Autodesk Inventor part; units mm, degrees
ref_plane "YZ Plane" through (0, 0, 0) normal (1, 0, 0) x (0, 1, 0)
ref_plane "XZ Plane" through (0, 0, 0) normal (0, 1, 0) x (-1, 0, 0)
ref_plane "XY Plane" through (0, 0, 0) normal (0, 0, 1) x (1, 0, 0)
sketch "Sketch2" plane through (0, 0, 0) normal (0, 0, 1) x (1, 0, 0)
  line L0 (-36.8686, 26.7016) -> (-30.1114, 30.7457)
  line L1 (-30.1114, 30.7457) -> (-23.2304, 26.9158)
  line L2 (-23.2304, 26.9158) -> (-23.1068, 19.0418)
  line L3 (-23.1068, 19.0418) -> (-29.864, 14.9977)
  line L4 (-29.864, 14.9977) -> (-36.7449, 18.8276)
  line L5 (-36.7449, 18.8276) -> (-36.8686, 26.7016)
  line L6 (-111.0137, 35.5717) -> (-17.2877, 35.5717)
  line L7 (-17.2877, 35.5717) -> (-17.2877, -24.1183)
  line L8 (-17.2877, -24.1183) -> (-111.0137, -24.1183)
  line L9 (-111.0137, -24.1183) -> (-111.0137, 35.5717)
  line L10 (-101.137, 28.7391) -> (-70.6621, 28.7391)
  line L11 (-70.6621, 28.7391) -> (-70.6621, -18.2509)
  line L12 (-70.6621, -18.2509) -> (-101.137, -18.2509)
  line L13 (-101.137, -18.2509) -> (-101.137, 28.7391)
  point P0 (0, 0)
  point P1 (-29.9877, 22.8717)
  dimension "d1" = 7.874
  dimension "d3" = 59.69
  dimension "d5" = 12.7
  dimension "d6" = 93.726
  dimension "d39" = 46.99
  dimension "d41" = 6.8326
  dimension "d42" = 5.8674
  dimension "d43" = 12.7
extrude "Extrusion1" add sketch "Sketch2" along normal blind 6.35 contours L6 L7 L8 L9 | L10 L11 L12 L13
sketch "Sketch3" plane through (0, 0, 6.35) normal (0, 0, 1) x (1, 0, 0)
  circle A0 centre (-107.8387, 30.4917) radius 1.905
  line L0 (-17.2877, 35.5717) -> (-111.0137, 35.5717)
  line L1 (-111.0137, 35.5717) -> (-111.0137, -24.1183)
  circle A1 centre (-107.8387, 20.3317) radius 1.905
  circle A2 centre (-107.8387, -10.1483) radius 1.905
  circle A3 centre (-107.8387, -20.3083) radius 1.905
  line L2 (-111.0137, -24.1183) -> (-17.2877, -24.1183)
  circle A4 centre (-107.8387, 10.1717) radius 1.905
  circle A5 centre (-107.8387, 0.0117) radius 1.905
  point P0 (0, 0)
  dimension "d9" = 3.81
  dimension "d10" = 5.08
  dimension "d11" = 3.175
  dimension "d13" = 3.81
  dimension "d14" = 3.81
  dimension "d15" = 3.81
  dimension "d17" = 3.175
  dimension "d18" = 3.175
  dimension "d19" = 3.175
  dimension "d21" = 10.16
  dimension "d24" = 3.81
  dimension "d25" = 3.81
  dimension "d26" = 3.175
  dimension "d27" = 3.175
  dimension "d28" = 10.16
  dimension "d29" = 10.16
  dimension "d33" = 10.16
  dimension "d44" = 10.16
extrude "Extrusion2" cut sketch "Sketch3" against normal blind 3.81
sketch "Sketch4" plane through (0, 0, 6.35) normal (0, 0, 1) x (1, 0, 0)
  line L0 (-17.2877, 35.5717) -> (-111.0137, 35.5717)
  line L1 (-72.9137, 35.5717) -> (-60.2137, 35.5717)
  line L2 (-60.2137, 35.5717) -> (-60.2137, 35.0891)
  line L3 (-60.2137, 35.0891) -> (-72.9137, 35.0891)
  line L4 (-72.9137, 35.0891) -> (-72.9137, 35.5717)
  line L5 (-111.0137, -24.1183) -> (-17.2877, -24.1183)
  line L6 (-111.0137, 35.5717) -> (-111.0137, -24.1183)
  line L7 (-72.9137, 35.5717) -> (-60.2137, 35.5717)
  line L8 (-60.2137, 35.5717) -> (-60.2137, 28.7391)
  line L9 (-60.2137, 28.7391) -> (-72.9137, 28.7391)
  line L10 (-72.9137, 28.7391) -> (-72.9137, 35.5717)
  line L11 (-69.1037, -24.1183) -> (-81.8037, -24.1183)
  line L12 (-81.8037, -24.1183) -> (-81.8037, -18.1493)
  line L13 (-81.8037, -18.1493) -> (-69.1037, -18.1493)
  line L14 (-69.1037, -18.1493) -> (-69.1037, -24.1183)
  point P0 (0, 0)
  dimension "d34" = 59.2074
  dimension "d35" = 12.7
  dimension "d36" = 38.1
  dimension "d45" = 6.8326
  dimension "d46" = 12.7
  dimension "d47" = 5.969
  dimension "d48" = 29.21
extrude "Extrusion3" add sketch "Sketch4" along normal blind 6.35
properties part number "polyhexpart"
Could you check a few things on this model? Use its own coordinates, in mm. A direction names the side the tool comes from. Round coordinates to 2 decimals unless told otherwise and drop trailing zeros. Write each loop counter-clockwise with the first axis right and the second up, starting at its lowest first coordinate (ties: lowest second). Pieces come first, ordered by that corner, then holes. Notation, with made-up numbers: M 69,27 L 104,27 A15 ccw 104,33 Z; hole C 0,-15.75 d5. An arc over 180 degrees is marked long. Answer in a Markdown table with one row per item. Add a question column.
Q1. Imagine slicing it at B-B (x = -70.5). Please give me the cut outline in (y, z).
Q2. Will these pins go through, and if not, where does the flat tip stop? pin 1 Ø3 at (x, y) = (-34.5, 18.5) entering from +Z; pin 2 Ø4.5 at (x, y) = (-107.84, -20.31) entering from -Z; pin 3 Ø7 at (x, z) = (-64.5, 10.5) entering from -Y; pin 4 Ø1.9 at (x, y) = (-108, -11) entering from +Z.
Q3. Imagine slicing it at D-D (z = 3.5). Please give me the cut outline in (x, y) (3 decimals), then the cut area to 3 significant figures.
Q4. Imagine slicing it at C-C (x = -25). Please give me the cut outline in (y, z), then the cut area to 3 significant figures.
Q5. On a 3-axis mill with a long thin cutter (end or side, diameter ignored), from which of +Z, -Z, +X, -X, +Y, -Y can I reach the whole of each face in a straight line? I mean faces 1 (the flat face through (-69.104, -21, 9)), 2 (the cylindrical face through (-106.02, 10.74, 4.47)), 3 (the flat face through (-76, -18.149, 9)). Say none if no direction works.
Q6. If I drill on line 1 (X direction, y = 10, z = 5.5); line 2 (X direction, y = 25.5, z = 3.25); line 3 (X direction, y = 20, z = 3), over which ranges is the centre line in solid material (lowest first)? Write a range as from..to.
Q7. Imagine slicing it at A-A (z = 8.25). Please give me the cut outline in (x, y).
Q8. If we mould it in two halves opening along Y, with no side actions, what happens to faces 4 (the flat face through (-65, 35.572, 3)), 5 (the flat face through (-108, 0, 2.54)), 6 (the flat face through (-72.914, 32, 9))? For each: +Y half, -Y half, draft (parallel to the pull), parting line (faces both ways), or undercut.
Values:
| question | item | result |
|---|---|---|
| 1 | outline | M -24.12,0 L 35.57,0 L 35.57,12.7 L 28.74,12.7 L 28.74,6.35 L -18.15,6.35 L -18.15,12.7 L -24.12,12.7 Z |
| 2 | pin 1 | z = 6.35 |
| 2 | pin 2 | z = 0 |
| 2 | pin 3 | y = 28.74 |
| 2 | pin 4 | z = 2.54 |
| 3 | outline | M -111.014,-24.118 L -17.288,-24.118 L -17.288,35.572 L -111.014,35.572 Z; hole C -107.839,-20.308 d3.81; hole C -107.839,-10.148 d3.81; hole C -107.839,0.012 d3.81; hole C -107.839,10.172 d3.81; hole C -107.839,20.332 d3.81; hole C -107.839,30.492 d3.81; hole M -36.869,26.702 L -36.745,18.828 L -29.864,14.998 L -23.107,19.042 L -23.23,26.916 L -30.111,30.746 Z |
| 3 | area | 5,360 mm^2 |
| 4 | outline | M -24.12,0 L 17.91,0 L 17.91,6.35 L -24.12,6.35 Z; M 27.9,0 L 35.57,0 L 35.57,6.35 L 27.9,6.35 Z |
| 4 | area | 316 mm^2 |
| 5 | face 1 | +Z, +X, -Y |
| 5 | face 2 | +Z |
| 5 | face 3 | +Z, +X, -X |
| 6 | line 1 | -111.01..-109.74, -105.94..-17.29 |
| 6 | line 2 | -111.01..-36.85, -23.21..-17.29 |
| 6 | line 3 | -111.01..-109.71, -105.96..-36.76, -23.12..-17.29 |
| 7 | outline | M -81.8,-24.12 L -69.1,-24.12 L -69.1,-18.15 L -81.8,-18.15 Z; M -72.91,28.74 L -60.21,28.74 L -60.21,35.57 L -72.91,35.57 Z |
| 8 | face 4 | +Y half |
| 8 | face 5 | undercut |
| 8 | face 6 | draft |
